```python
from build123d import *

# Parameters (mm, degrees)
RESSALTO_EXTRUS_O1_DEPTH = 20
CASCA1_T                 = -1.5
ESBO_O2_R                = 1.5
RESSALTO_EXTRUS_O2_DEPTH = 30


with BuildPart() as part:
    # Esboço1 → Ressalto-extrusão1 (new body)
    with BuildSketch(Plane.XY):
        Polygon((-12.986930378, 8.7142726), (-15.044163089, 4.274583549), (-15.628768299, -0.583531522), (-14.683520775, -5.384526462), (-12.300947932, -9.658446435), (-8.7142726, -12.986930378), (-4.274583549, -15.044163089), (0.583531522, -15.628768299), (5.384526462, -14.683520775), (9.658446435, -12.300947932), (12.986930378, -8.7142726), (15.044163089, -4.274583549), (15.628768299, 0.583531522), (14.683520775, 5.384526462), (12.300947932, 9.658446435), (8.7142726, 12.986930378), (4.274583549, 15.044163089), (-0.583531522, 15.628768299), (-5.384526462, 14.683520775), (-9.658446435, 12.300947932), align=None)
    extrude(amount=RESSALTO_EXTRUS_O1_DEPTH)

    # Casca1
    casca1_openings = [part.faces().sort_by_distance(p)[0] for p in [
        (0, 0, 0),
    ]]
    offset(amount=CASCA1_T, openings=casca1_openings, kind=Kind.INTERSECTION)

    # Esboço2 → Ressalto-extrusão2 (add)
    with BuildSketch(Plane.XY.offset(20)):
        Circle(ESBO_O2_R)
    extrude(amount=RESSALTO_EXTRUS_O2_DEPTH)


solid = part.part
```
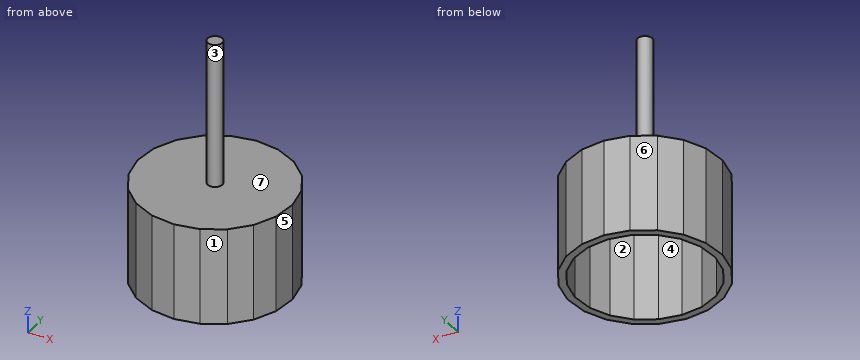
The listing builds one solid part. Answer for the finished solid, in the listing's coordinates (mm). Face numbers are marked on the shaded views. A direction names the side the tool comes from. Round coordinates to 2 decimals unless told otherwise and drop trailing zeros. Loops run counter-clockwise (first coordinate to the right, second up) from the corner with the lowest first, then second, coordinate; pieces in that order, holes last.
1) A cutting plane is placed at A-A on y = -10.5. Determine the outline of the cut face in (x, z).
Outcome:
outline: (-11.39, 0) - (-9.19, 0) - (-9.19, 18.5) - (9.28, 18.5) - (9.28, 0) - (11.33, 0) - (11.33, 20) - (-11.39, 20) - close
2) A cutting plane is placed at C-C on z = 43. Determine the outline of the cut face in (x, y), plus the area to 3 significant figures.
Outcome:
outline: circle Ø3 at (0, 0)
area: 7.07 mm2
3) Consider line 1 (Z direction, x = 10, y = 4); line 2 (Z direction, x = 8, y = -12); line 3 (Y direction, x = 3, z = 2). Determine where each line is inside the solid, lowest interval first.
Outcome:
line 1: z = 18.5 to 20
line 2: z = 0 to 20
line 3: y = -15.15 to -13.62, 13.69 to 15.2
4) A cutting plane is placed at B-B on x = -6.5. Determine the outline of the cut face in (y, z), plus the area to 3 significant figures.
Outcome:
outline: (-14.01, 0) - (-12.36, 0) - (-12.36, 18.5) - (12.34, 18.5) - (12.34, 0) - (14.06, 0) - (14.06, 20) - (-14.01, 20) - close
area: 104 mm2
5) For the marked faces 1, 2 and 3, determine the directions among +Z, -Z, +X, -X, +Y, -Y from which every point of the face is accessible in a straight line to the end or side of a thin tool.
Outcome:
face 1: +Z, -Z, +X, -Y
face 2: -Z
face 3: +Z
6) Given P1, Ø1, axis at x = -11, y = -3.5, coming from the -Z side; P2, Ø3, axis at x = 0, z = 32, coming from the +Y side; P3, Ø4, axis at y = 2, z = 29.5, coming from the +X side, each flat-ended and moving along its own axis, determine where each tip first touches the part or whether it passes through.
Outcome:
P1: stops at z = 18.5
P2: stops at y = 1.5
P3: stops at x = 1.5
7) For a pull along Y with two mould halves and no side action, classify the marked faces 4, 5, 6 and 7 as released by +Y, released by -Y, zero draft, split by the parting line, or undercut.
Outcome:
face 4: undercut
face 5: released by -Y
face 6: released by +Y
face 7: zero draft
